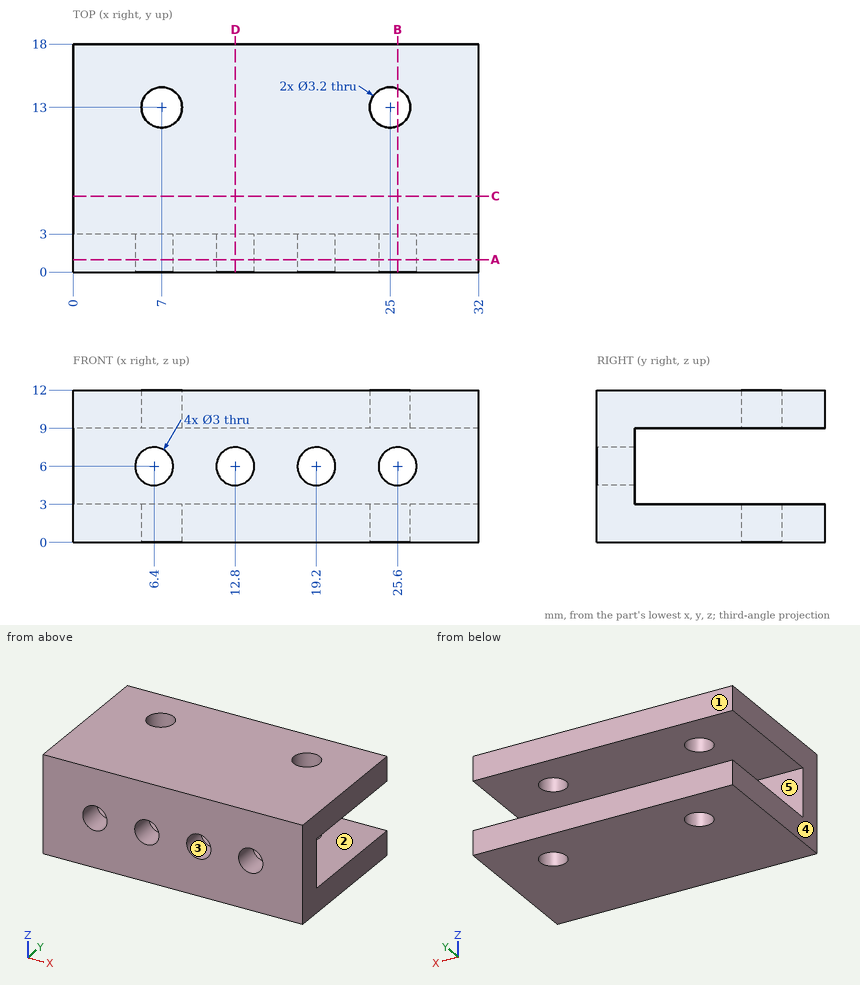
Input: dimensioned drawing with shaded views. Units: mm. Origin: part minimum x, y, z. A direction names the side the tool comes from. Give positions to 0.01 mm unless a question says otherwise; leave off trailing zeros. Write each loop counter-clockwise with the first axis right and the second up, starting at its lowest first coordinate (ties: lowest second). Pieces come first, ordered by that corner, then holes. Notation, with made-up numbers: M 15.5,36.5 L 30.5,36.5 A10 ccw 30.5,44.5 Z; hole C 41,40.5 d11. An arc over 180 degrees is marked long. Return JSON: item names as keys, results as strings. Group by question number.
1) Cut plane D-D, the plane x = 12.8. Output: boundary loops of the cut face in (y, z).
2) Cut plane C-C, the plane y = 6. Output: boundary loops of the cut face in (x, z).
3) Pull-direction query (X, two-part tool) for the marked faces 3, 4 and 5; classes: pulls with the +X half, pulls with the -X half, needs draft (parallel to the pull), parting line crosses it, or undercut.
4) Set-up query: the marked faces 1 and 2. Return all of +Z, -Z, +X, -X, +Y, -Y with unobstructed straight access to the full face (end or side cutting, diameter ignored); none if empty.
5) Material intervals for line 1 along Z through (x, y) = (21, 9.25); line 2 along X through (y, z) = (13, 1.15); line 3 along Z through (x, y) = (19.2, 0.95), sorted ascending. Write a range as [from, to].
6) Cut plane B-B, the plane x = 25.6. Output: boundary loops of the cut face in (y, z), plus the area to 3 significant figures.
7) Cut plane A-A, the plane y = 1. Output: boundary loops of the cut face in (x, z), plus the area to 3 significant figures.
Recorded:
{
 "1": {"outline": "M 0,0 L 18,0 L 18,3 L 3,3 L 3,4.5 L 0,4.5 Z; M 0,7.5 L 3,7.5 L 3,9 L 18,9 L 18,12 L 0,12 Z"},
 "2": {"outline": "M 0,0 L 32,0 L 32,3 L 0,3 Z; M 0,9 L 32,9 L 32,12 L 0,12 Z"},
 "3": {"face 3": "undercut", "face 4": "pulls with the -X half", "face 5": "needs draft"},
 "4": {"face 1": "+Z, -Z, +X, -X, +Y", "face 2": "+X, -X, +Y"},
 "5": {"line 1": "z = [0, 3], [9, 12]", "line 2": "x = [0, 5.4], [8.6, 23.4], [26.6, 32]", "line 3": "z = [0, 4.5], [7.5, 12]"},
 "6": {"outline": "M 0,0 L 11.52,0 L 11.52,3 L 3,3 L 3,4.5 L 0,4.5 Z; M 0,7.5 L 3,7.5 L 3,9 L 11.52,9 L 11.52,12 L 0,12 Z; M 14.48,0 L 18,0 L 18,3 L 14.48,3 Z; M 14.48,9 L 18,9 L 18,12 L 14.48,12 Z", "area": "99.2 mm²"},
 "7": {"outline": "M 0,0 L 32,0 L 32,12 L 0,12 Z; hole C 6.4,6 d3; hole C 12.8,6 d3; hole C 19.2,6 d3; hole C 25.6,6 d3", "area": "356 mm²"}
}
